Check sheet for the drawn part. Datum: minimum x, y, z corner. Units: mm. Give positions to 0.01 mm unless a question says otherwise; leave off trailing zeros. Write each loop counter-clockwise with the first axis right and the second up, starting at its lowest first coordinate (ties: lowest second). Pieces come first, ordered by that corner, then holes. Notation, with made-up numbers: (27.5, -12.5) -> (48.5, -12.5) arc R8 ccw to (48.5, -5.5) -> close; hole circle Ø4 at (17, 18). An arc over 180 degrees is marked (long way). Answer as CSV lines item,"result". Start each with the question number.
1) Gauge pin test, flat ends, axial feed: pin 1 Ø0.5 at (x, y) = (1, 7.5) entering from -Z (3 decimals); pin 2 Ø0.7 at (x, y) = (1.5, 2) entering from +Z (3 decimals); pin 3 Ø0.5 at (y, z) = (8.5, 1) entering from +X (3 decimals). Record the tip position at first contact, or that the pin passes through.
2) Material ranges on L1, parallel to Y at x = 2.1, z = 1; L2, parallel to X at y = 7.5, z = 1.2 (3 decimals); L3, parallel to Z at x = 1.1, y = 6 (3 decimals), recorded low to high.
3) Mould release check, pull along Z, two halves, no side actions. Record for the marked faces 1, 2, 3 and 4: released by +Z, released by -Z, zero draft, split by the parting line, or undercut.
4) Sectioned sample at D-D on y = 0.5. Record the cut outline in (x, z) (3 decimals).
5) Sectioned sample at B-B on x = 2.15. Record the cut outline in (y, z), and give its area (3 significant figures).
6) Sectioned sample at A-A on y = 4. Record the cut outline in (x, z).
7) Sectioned sample at C-C on z = 0.4. Record the cut outline in (x, y), and give its area (3 significant figures).
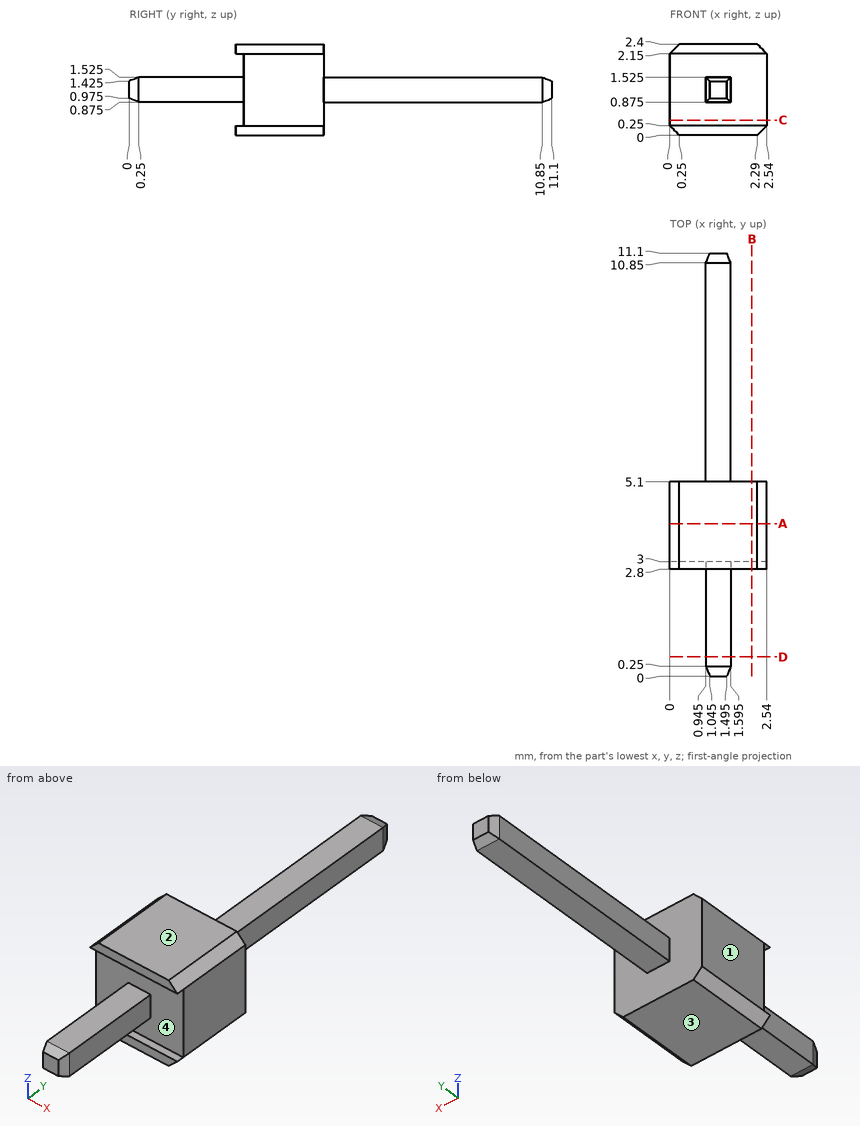
Ans:
1,pin 1,"stops at z = 0.875"
1,pin 2,"stops at z = 1.525"
1,pin 3,"stops at x = 1.595"
2,L1,"y = 3 to 5.1"
2,L2,"x = 0.945 to 1.595"
2,L3,"z = 0.875 to 1.525"
3,face 1,"zero draft"
3,face 2,"released by +Z"
3,face 3,"released by -Z"
3,face 4,"undercut"
4,outline,"(0.945, 0.875) -> (1.595, 0.875) -> (1.595, 1.525) -> (0.945, 1.525) -> close"
5,outline,"(2.8, 0) -> (5.1, 0) -> (5.1, 2.4) -> (2.8, 2.4) -> (2.8, 2.15) -> (3, 2.15) -> (3, 0.25) -> (2.8, 0.25) -> close"
5,area,"5.14 mm²"
6,outline,"(0, 0.25) -> (0.25, 0) -> (2.29, 0) -> (2.54, 0.25) -> (2.54, 2.15) -> (2.29, 2.4) -> (0.25, 2.4) -> (0, 2.15) -> close"
7,outline,"(0, 3) -> (2.54, 3) -> (2.54, 5.1) -> (0, 5.1) -> close"
7,area,"5.33 mm²"
